from build123d import *

# Parameters (mm, degrees)
BOSS_EXTRUDE1_DEPTH         = 10
SKETCH2_R                   = 1
CUT_EXTRUDE1_DEPTH          = 0.6
SKETCH3_R                   = 1.99
SKETCH3_R_2                 = 2
BOSS_EXTRUDE3_DEPTH         = 8
CHAMFER3_SIZE               = 1
HOLE_WIZARD_M31_D           = 3.2
HOLE_WIZARD_M31_CSINK_D     = 6.3
HOLE_WIZARD_M31_CSINK_ANGLE = 90
M3X0_51_D                   = 2.5
M3X0_51_DEPTH               = 6.5
M3X0_51_TIP                 = 0.751075774


with BuildPart() as part:
    # Sketch1 → Boss-Extrude1 (new body)
    with BuildSketch(Plane.XY):
        with BuildLine():
            Line((-12, -36), (12, -36))
            Line((12, -36), (12, 10))
            ThreePointArc((12, 10), (11.414213562, 11.414213562), (10, 12))
            Line((10, 12), (-10, 12))
            ThreePointArc((-10, 12), (-11.414213562, 11.414213562), (-12, 10))
            Line((-12, 10), (-12, -36))
        make_face()
    extrude(amount=BOSS_EXTRUDE1_DEPTH)

    # Sketch2 → Cut-Extrude1 (cut)
    with BuildSketch(Plane(origin=(0, 0, 0), x_dir=(-1, 0, 0), z_dir=(0, 0, -1))):
        with Locations((4, -8)):
            Circle(SKETCH2_R)
        with Locations((-0.116, -14.973)):
            Circle(SKETCH2_R)
        with BuildLine():
            Line((-1, -1.5), (1, -1.5))
            ThreePointArc((1, -1.5), (1.853553391, -1.853553391), (1.5, -1))
            Line((1.5, -1), (1.5, 1))
            ThreePointArc((1.5, 1), (1.853553391, 1.853553391), (1, 1.5))
            Line((1, 1.5), (-1, 1.5))
            ThreePointArc((-1, 1.5), (-1.853553391, 1.853553391), (-1.5, 1))
            Line((-1.5, 1), (-1.5, -1))
            ThreePointArc((-1.5, -1), (-1.853553391, -1.853553391), (-1, -1.5))
        make_face()
        with BuildLine():
            Line((-1.76, -26.26), (1.76, -26.26))
            ThreePointArc((1.76, -26.26), (2.613553391, -26.613553391), (2.26, -25.76))
            Line((2.26, -25.76), (2.26, -22.24))
            ThreePointArc((2.26, -22.24), (2.613553391, -21.386446609), (1.76, -21.74))
            Line((1.76, -21.74), (-1.76, -21.74))
            ThreePointArc((-1.76, -21.74), (-2.613553391, -21.386446609), (-2.26, -22.24))
            Line((-2.26, -22.24), (-2.26, -25.76))
            ThreePointArc((-2.26, -25.76), (-2.613553391, -26.613553391), (-1.76, -26.26))
        make_face()
    extrude(amount=-CUT_EXTRUDE1_DEPTH, mode=Mode.SUBTRACT)

    # Sketch3 → Boss-Extrude3 (add)
    with BuildSketch(Plane.XY.offset(10)):
        Circle(SKETCH3_R)
        with Locations((0, -24)):
            Circle(SKETCH3_R_2)
    extrude(amount=BOSS_EXTRUDE3_DEPTH)

    # Chamfer3
    chamfer3_edges = [part.edges().sort_by_distance(p)[0] for p in [
        (-1.99, 0, 18),
        (-2, -24, 18),
    ]]
    chamfer(chamfer3_edges, length=CHAMFER3_SIZE)

    # Зенковка для  винта с полупотайной головкой M31 (through all)
    with Locations(Plane(origin=(0, 0, 0), x_dir=(-1, 0, 0), z_dir=(0, 0, -1))):
        with Locations((6, 0), (-6, 0), (-6, -24), (6, -24)):
            CounterSinkHole(HOLE_WIZARD_M31_D / 2, HOLE_WIZARD_M31_CSINK_D / 2, counter_sink_angle=HOLE_WIZARD_M31_CSINK_ANGLE)

    # Отверстие обработанное метчиком M3x0.51
    with Locations(Plane(origin=(0, 0, 0), x_dir=(-1, 0, 0), z_dir=(0, 0, -1))):
        with Locations((-6.5, -8), (-6.5, 9), (7.5, 9), (7.5, -8), (6.884, -14.975), (6.884, -31.973), (-7.116, -14.973), (-7.116, -31.973)):
            Hole(M3X0_51_D / 2, depth=M3X0_51_DEPTH)
            with Locations((0, 0, -(M3X0_51_DEPTH + M3X0_51_TIP / 2))):  # 118° drill point
                Cone(0, M3X0_51_D / 2, M3X0_51_TIP, mode=Mode.SUBTRACT)


solid = part.part
Read the model definition and answer for the solid it produces. Units are mm, in the model's axes. A direction names the side the tool comes from. Round coordinates to 2 decimals unless told otherwise and drop trailing zeros. Loops run counter-clockwise (first coordinate to the right, second up) from the corner with the lowest first, then second, coordinate; pieces in that order, holes last. Notation, with made-up numbers: (-34.5, 50.5) - (-13.5, 50.5) arc R22 ccw to (-13.5, 88.5) - close; hole circle Ø2 at (-25, -21.75). An arc over 180 degrees is marked (long way). One line per question, with ' | ' between items. Start each with the question number.
Q1. Section A-A on z = 13.5 is taken. Give the vertices of the cut face in (x, y).
Q2. For a pull along X with two mould halves and no side action, classify faces 4 (the flat face through (12, -13, 5)), 5 (the conical face through (7.14, -31.76, 7.12)), 6 (the flat face through (0, -12, 0)), 7 (the cylindrical face through (2.625, -26.602, 0.296)) as +X half, -X half, draft (parallel to the pull), parting line (faces both ways), or undercut.
Q3. Flat-ended cylindrical pins translate along their axes: pin 1 (0.6 mm diameter, centred on x = 2.26, y = -21.74, fed in from +Z); pin 2 (1.9 mm diameter, centred on x = -6, y = 0, fed in from -Z); pin 3 (1.5 mm diameter, centred on x = -6.884, y = -31.973, fed in from -Z); pin 4 (1.2 mm diameter, centred on x = -4, y = -8, fed in from -Z). Find the tip coordinate at first contact, or state that the pin passes through.
Q4. Section C-C on y = -28.5 is taken. Give the vertices of the cut face in (x, z), plus the area to 3 significant figures.
Q5. For faces 1 (the flat face through (0, 0, 18)), 2 (the cylindrical face through (0, -22, 13)), 3 (the cylindrical face through (0.33, -15.95, 0.3)), determine the directions among +Z, -Z, +X, -X, +Y, -Y from which every point of the face is accessible in a straight line to the end or side of a thin tool.
Q6. Find the intervals of material crossed by L1, parallel to X at y = 9, z = 5.25; L2, parallel to Y at x = -6, z = 6; L3, parallel to X at y = -8.5, z = 6.25, in increasing order.
Q7. Section B-B on z = 2.5 is taken. Count the separate pieces of the cut face and the enclosed holes in it, plus the area to 3 significant figures.
Established:
1) outline: circle Ø4 at (0, -24); circle Ø3.98 at (0, 0)
2) face 4: +X half | face 5: undercut | face 6: draft | face 7: undercut
3) pin 1: z = 10 | pin 2: through | pin 3: z = 6.8 | pin 4: z = 0.6
4) outline: (-12, 0) - (12, 0) - (12, 10) - (-12, 10) - close | area: 240 mm²
5) face 1: +Z, +X, -X, +Y, -Y | face 2: +Z | face 3: -Z
6) L1: -12 to -8.75, -6.25 to 5.25, 7.75 to 12 | L2: -36 to -32.86, -31.09 to -25.6, -22.4 to -15.86, -14.09 to -1.6, 1.6 to 12 | L3: -12 to -8.65, -6.35 to 5.35, 7.65 to 12
7) separate pieces: 1 | enclosed holes: 12 | area: 1,080 mm²
